Input: part model. Units: mm. Frame: model coordinates. Give positions to 0.01 mm unless a question says otherwise; leave off trailing zeros. Loops run counter-clockwise (first coordinate to the right, second up) from the corner with the lowest first, then second, coordinate; pieces in that order, holes last. Notation, with made-up numbers: (49.5, -17) -> (59.5, -17) arc R20 cw to (59.5, -2) -> close; hole circle Ø8 at (-20.5, 56). An arc over 180 degrees is marked (long way). One line per question, with ' | ' between items.
from build123d import *

# Parameters (mm, degrees)
F0_W     = 38.1
F0_H     = 38.1
F0_W_2   = 33.8836
F0_H_2   = 33.8836
F1_DEPTH = 431.8
F2_W     = 38.1
F2_H     = 12.7
F3_DEPTH = 0.254
F4_R     = 3.175
F5_DEPTH = 76.2


with BuildPart() as f1:
    # F0 (on Front) → F1 (new body)
    with BuildSketch(Plane.XZ):
        with Locations((-45.121367, 19.295737)):
            Rectangle(F0_W, F0_H)
        with Locations((-45.121367, 19.295737)):
            Rectangle(F0_W_2, F0_H_2, mode=Mode.SUBTRACT)
    extrude(amount=F1_DEPTH)

    # F2 (on face) → F3 (join)
    with BuildSketch(Plane(origin=(0, 0, 0.245737), x_dir=(1, 0, 0), z_dir=(0, 0, -1))):
        with Locations((-45.121367, 31.75)):
            Rectangle(F2_W, F2_H)
    extrude(amount=F3_DEPTH)

    # F4 (on face) → F5 (cut)
    with BuildSketch(Plane(origin=(0, 0, 0.245737), x_dir=(1, 0, 0), z_dir=(0, 0, -1))):
        with Locations((-45.121367, 333.375)):
            Circle(F4_R)
    extrude(amount=-F5_DEPTH, mode=Mode.SUBTRACT)


solid = f1.part
1. Pin query (flat end, axial travel): P1, Ø12.5, axis at x = -52, y = -18, coming from the -Z side; P2, Ø5.5, axis at x = -45.12, y = -333.38, coming from the +Z side. Return the tip coordinate at first contact, or that it passes through.
Determined:
P1: stops at z = 0.25 | P2: passes through
2. Pull-direction query (Z, two-part tool) for faces 1 (the flat face through (-45, -232, 0.246)), 2 (the flat face through (-45, -213, 38.346)), 3 (the flat face through (-45, -213, 36.238)), 4 (the flat face through (-45, -213, 2.354)); classes: pulls with the +Z half, pulls with the -Z half, needs draft (parallel to the pull), parting line crosses it, or undercut.
Determined:
face 1: pulls with the -Z half | face 2: pulls with the +Z half | face 3: undercut | face 4: undercut
3. Section query B-B (x = -32). Output: boundary loops of the cut face in (y, z), then the cut area to 3 significant figures.
Determined:
outline: (-431.8, 0.25) -> (-38.1, 0.25) -> (-38.1, -0.01) -> (-25.4, -0.01) -> (-25.4, 0.25) -> (0, 0.25) -> (0, 2.35) -> (-431.8, 2.35) -> close; (-431.8, 36.24) -> (0, 36.24) -> (0, 38.35) -> (-431.8, 38.35) -> close | area: 1,820 mm2
4. Section query A-A (z = 22). Output: boundary loops of the cut face in (x, y).
Determined:
outline: (-64.17, -431.8) -> (-62.06, -431.8) -> (-62.06, 0) -> (-64.17, 0) -> close; (-28.18, -431.8) -> (-26.07, -431.8) -> (-26.07, 0) -> (-28.18, 0) -> close
5. Section query C-C (y = -221.5). Output: boundary loops of the cut face in (x, z).
Determined:
outline: (-64.17, 0.25) -> (-26.07, 0.25) -> (-26.07, 38.35) -> (-64.17, 38.35) -> close; hole (-62.06, 2.35) -> (-28.18, 2.35) -> (-28.18, 36.24) -> (-62.06, 36.24) -> close
6. Ray query, line 1 along X through (y, z) = (-306, 33.5); line 2 along Z through (x, y) = (-28.5, -65). Return the intervals inside material, ascending. Write a range as from..to.
Determined:
line 1: x = -64.17..-62.06, -28.18..-26.07 | line 2: z = 0.25..2.35, 36.24..38.35
